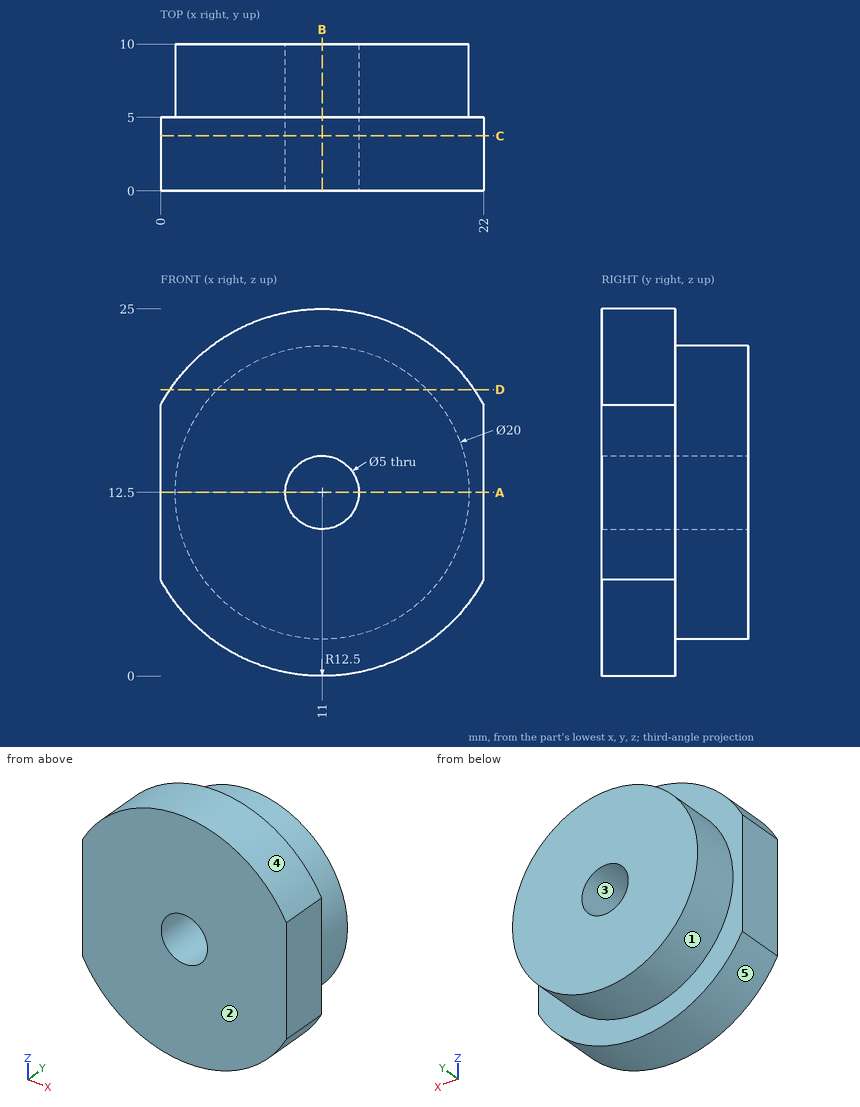
Geometry: see drawing. Coordinates: mm, zero at the bounding-box minimum. A direction names the side the tool comes from. Coordinates: 2 decimals unless noted, no trailing zeros. Order: outer loops, then holes, each group sorted by start corner. A loop starts at its lowest first (then second) coordinate and runs counter-clockwise, first axis right, second up. Notation, with made-up numbers: (17, -20) - (43, -20) arc R22 cw to (43, 14) - close; hole circle Ø9 at (70, -9.75). An arc over 180 degrees is marked (long way). Write each question's results on one line, items separated by ' | '.
(1) Line query: line 1 (X direction, y = 4, z = 12.5); line 2 (X direction, y = 4.5, z = 5); line 3 (Z direction, x = 9.5, y = 2.5). Output: solid intervals per line, ascending. Write a range as [from, to].
Values found:
line 1: x = [0, 8.5], [13.5, 22] | line 2: x = [1, 21] | line 3: z = [0.09, 10.5], [14.5, 24.91]
(2) Section query A-A, the plane z = 12.5. Return the cut outline in (x, y).
Values found:
outline: (0, 0) - (8.5, 0) - (8.5, 10) - (1, 10) - (1, 5) - (0, 5) - close; (13.5, 0) - (22, 0) - (22, 5) - (21, 5) - (21, 10) - (13.5, 10) - close
(3) First-contact query: pin 1 Ø6 at (x, z) = (11, 12.5) entering from -Y; pin 2 Ø1 at (x, y) = (6, 2.5) entering from +Z. Flat tips, straight axial feed; report the tip coordinate or a pass-through.
Values found:
pin 1: stops at y = 0 | pin 2: stops at z = 24.16
(4) Mould query, pull axis Z, two halves, no side actions, for the marked faces 3, 4 and 5. Classes: +Z half, -Z half, draft (parallel to the pull), parting line (faces both ways), or undercut.
Values found:
face 3: undercut | face 4: +Z half | face 5: -Z half
(5) Section query C-C, the plane y = 3.75. Return the cut outline in (x, z), plus the area to 3 significant figures.
Values found:
outline: (0, 6.56) arc R12.5 ccw to (22, 6.56) - (22, 18.44) arc R12.5 ccw to (0, 18.44) - close; hole circle Ø5 at (11, 12.5) | area: 447 mm²
(6) Section query D-D, the plane z = 19.5. Return the cut outline in (x, y).
Values found:
outline: (0.64, 0) - (21.36, 0) - (21.36, 5) - (18.14, 5) - (18.14, 10) - (3.86, 10) - (3.86, 5) - (0.64, 5) - close
(7) Section query B-B, the plane x = 11. Return the cut outline in (y, z).
Values found:
outline: (0, 0) - (5, 0) - (5, 2.5) - (10, 2.5) - (10, 10) - (0, 10) - close; (0, 15) - (10, 15) - (10, 22.5) - (5, 22.5) - (5, 25) - (0, 25) - close
(8) Set-up query: the marked faces 1 and 2. Return all of +Z, -Z, +X, -X, +Y, -Y with unobstructed straight access to the full face (end or side cutting, diameter ignored); none if empty.
Values found:
face 1: +Y | face 2: +Z, -Z, +X, -X, -Y
